Verification items for the finished model (mm, model axes). A direction names the side the tool comes from. Give positions to 0.01 mm unless a question says otherwise; leave off trailing zeros. Write each loop counter-clockwise with the first axis right and the second up, starting at its lowest first coordinate (ties: lowest second). Pieces come first, ordered by that corner, then holes.
from build123d import *
from build123d.topology import SkipClean

# Parameters (mm, degrees)
SKETCH1_R               = 19
BOSS_EXTRUDE1_DEPTH     = 5
BOSS_EXTRUDE4_DEPTH     = 20
SKETCH5_R               = 19
BOSS_EXTRUDE5_DEPTH     = 5
CUT_EXTRUDE1_DEPTH      = 37.701498607
CUT_EXTRUDE1_DEPTH_BACK = 5
SKETCH2_7_R             = 2.9
SKETCH1_3_R             = 9
CUT_EXTRUDE2_DEPTH      = 10
SKETCH6_R               = 2.5
BOSS_EXTRUDE7_DEPTH     = 25
FILLET1_R               = 5
SKETCH8_R               = 25
BOSS_EXTRUDE8_DEPTH     = 18


with BuildPart() as part:
    # Sketch1 → Boss-Extrude1 (new body)
    with BuildSketch(Plane(origin=(0, 0, 0), x_dir=(1, 0, 0), z_dir=(0, 1, 0))):
        with Locations(Location((0, 0, 0), (0, 0, 270))):
            Circle(SKETCH1_R)
    extrude(amount=BOSS_EXTRUDE1_DEPTH)

    # Sketch2 → Boss-Extrude4 (add)
    with SkipClean():  # the faces are left unmerged after this step: merging them gives an invalid solid
        with BuildSketch(Plane(origin=(0, 5, 0), x_dir=(1, 0, 0), z_dir=(0, 1, 0))):
            with BuildLine():
                Line((-14.008269399, 12.836213945), (-12.533714726, 11.485033529))
                ThreePointArc((-12.533714726, 11.485033529), (-12.02081528, 12.02081528), (-11.485033529, 12.533714726))
                Line((-11.485033529, 12.533714726), (-12.836213945, 14.008269399))
                ThreePointArc((-12.836213945, 14.008269399), (-13.435028843, 13.435028843), (-14.008269399, 12.836213945))
            make_face()
            with BuildLine():
                Line((14.008269399, 12.836213945), (12.533714726, 11.485033529))
                ThreePointArc((12.533714726, 11.485033529), (12.02081528, 12.02081528), (11.485033529, 12.533714726))
                Line((11.485033529, 12.533714726), (12.836213945, 14.008269399))
                ThreePointArc((12.836213945, 14.008269399), (13.435028843, 13.435028843), (14.008269399, 12.836213945))
            make_face()
            with BuildLine():
                Line((12.836213945, -14.008269399), (11.485033529, -12.533714726))
                ThreePointArc((11.485033529, -12.533714726), (12.02081528, -12.02081528), (12.533714726, -11.485033529))
                Line((12.533714726, -11.485033529), (14.008269399, -12.836213945))
                ThreePointArc((14.008269399, -12.836213945), (13.435028843, -13.435028843), (12.836213945, -14.008269399))
            make_face()
            with BuildLine():
                Line((-14.008269399, -12.836213945), (-12.533714726, -11.485033529))
                ThreePointArc((-12.533714726, -11.485033529), (-12.02081528, -12.02081528), (-11.485033529, -12.533714726))
                Line((-11.485033529, -12.533714726), (-12.836213945, -14.008269399))
                ThreePointArc((-12.836213945, -14.008269399), (-13.435028843, -13.435028843), (-14.008269399, -12.836213945))
            make_face()
        extrude(amount=BOSS_EXTRUDE4_DEPTH)

    # Sketch5 → Boss-Extrude5 (add)
    with SkipClean():  # the faces are left unmerged after this step: merging them gives an invalid solid
        with BuildSketch(Plane(origin=(0, 25, 0), x_dir=(1, 0, 0), z_dir=(0, 1, 0))):
            with Locations(Location((0, 0, 0), (0, 0, 270))):
                Circle(SKETCH5_R)
        extrude(amount=BOSS_EXTRUDE5_DEPTH)

    # Sketch2_7 → Cut-Extrude1 (cut, two sides: drawn at the far end of the back side and taken through both)
    with SkipClean():  # the faces are left unmerged after this step: merging them gives an invalid solid
        with BuildSketch(Plane(origin=(0, 5, 0), x_dir=(1, 0, 0), z_dir=(0, 1, 0)).offset(-CUT_EXTRUDE1_DEPTH_BACK)):
            with Locations(Location((14, 0, 0), (0, 0, 270))):
                Circle(SKETCH2_7_R)
            with Locations(Location((0, -14, 0), (0, 0, 270))):
                Circle(SKETCH2_7_R)
            with Locations(Location((0, 14, 0), (0, 0, 270))):
                Circle(SKETCH2_7_R)
            with Locations(Location((-14, 0, 0), (0, 0, 270))):
                Circle(SKETCH2_7_R)
        extrude(amount=CUT_EXTRUDE1_DEPTH + CUT_EXTRUDE1_DEPTH_BACK, mode=Mode.SUBTRACT)

    # Sketch1_3 → Cut-Extrude2 (cut)
    with SkipClean():  # the faces are left unmerged after this step: merging them gives an invalid solid
        with BuildSketch(Plane(origin=(0, 0, 0), x_dir=(1, 0, 0), z_dir=(0, 1, 0))):
            with Locations(Location((0, 0, 0), (0, 0, 270))):
                Circle(SKETCH1_3_R)
        extrude(amount=CUT_EXTRUDE2_DEPTH, mode=Mode.SUBTRACT)

    # Sketch6 → Boss-Extrude7 (add)
    with SkipClean():  # the faces are left unmerged after this step: merging them gives an invalid solid
        with BuildSketch(Plane(origin=(0, 30, 0), x_dir=(1, 0, 0), z_dir=(0, 1, 0))):
            with Locations(Location((0, 0, 0), (0, 0, 270))):
                Circle(SKETCH6_R)
        extrude(amount=BOSS_EXTRUDE7_DEPTH)

    # Fillet1
    fillet1_edges = [part.edges().sort_by_distance(p)[0] for p in [
        (0, 30, -2.5),
    ]]
    fillet(fillet1_edges, radius=FILLET1_R)

    # Sketch8 → Boss-Extrude8 (add)
    with SkipClean():  # the faces are left unmerged after this step: merging them gives an invalid solid
        with BuildSketch(Plane(origin=(0, 55, 0), x_dir=(1, 0, 0), z_dir=(0, 1, 0))):
            with Locations(Location((0, 0, 0), (0, 0, 270))):
                Circle(SKETCH8_R)
        extrude(amount=-BOSS_EXTRUDE8_DEPTH)


solid = part.part
Item 1: Sectioned sample at C-C on z = 16. Record the cut outline in (x, y).
Answer key:
outline: (-19.21, 37) - (19.21, 37) - (19.21, 55) - (-19.21, 55) - close; (-10.25, 0) - (-2.1, 0) - (-2.1, 5) - (-10.25, 5) - close; (-10.25, 25) - (-2.1, 25) - (-2.1, 30) - (-10.25, 30) - close; (2.1, 0) - (10.25, 0) - (10.25, 5) - (2.1, 5) - close; (2.1, 25) - (10.25, 25) - (10.25, 30) - (2.1, 30) - close
Item 2: Sectioned sample at B-B on y = 23.5. Record the cut outline in (x, z), then the cut area to 3 significant figures.
Answer key:
outline: (-14.01, -12.84) arc R19 ccw to (-12.84, -14.01) - (-11.49, -12.53) arc R17 cw to (-12.53, -11.49) - close; (-14.01, 12.84) - (-12.53, 11.49) arc R17 cw to (-11.49, 12.53) - (-12.84, 14.01) arc R19 ccw to start; (11.49, -12.53) - (12.84, -14.01) arc R19 ccw to (14.01, -12.84) - (12.53, -11.49) arc R17 cw to start; (11.49, 12.53) arc R17 cw to (12.53, 11.49) - (14.01, 12.84) arc R19 ccw to (12.84, 14.01) - close
area: 12.6 mm2
Item 3: Release check for a two-part mould opening along Z. For faces 1 (the face through (0.1, 2.5, -16.9)), 2 (the face through (-8, 30, 0)), 3 (the face through (12.17, 14.86, 13.28)), 4 (the face through (-13.28, 14.86, -12.17)) record: released by +Z, released by -Z, zero draft, split by the parting line, or undercut.
Answer key:
face 1: undercut
face 2: zero draft
face 3: released by +Z
face 4: undercut
Item 4: Sectioned sample at A-A on x = -15. Record the cut outline in (y, z).
Answer key:
outline: (0, -11.66) - (5, -11.66) - (5, -2.72) - (0, -2.72) - close; (0, 2.72) - (5, 2.72) - (5, 11.66) - (0, 11.66) - close; (25, -11.66) - (30, -11.66) - (30, -2.72) - (25, -2.72) - close; (25, 2.72) - (30, 2.72) - (30, 11.66) - (25, 11.66) - close; (37, -20) - (55, -20) - (55, 20) - (37, 20) - close
Item 5: Depth check by flat-ended pin: pin 1 (6 mm diameter, centred on y = 21, z = 2.5, fed in from +X); pin 2 (8 mm diameter, centred on y = 39.5, z = -14, fed in from -X); pin 3 (4.5 mm diameter, centred on x = 0, z = -14, fed in from -Y); pin 4 (1 mm diameter, centred on x = 16.5, y = 38, fed in from +Z). Enter the tip coordinate at first touch or a pass-through.
Answer key:
pin 1: passes through
pin 2: stops at x = -22.91
pin 3: stops at y = 37
pin 4: stops at z = 19.21
Item 6: Scan lines: line 1 along Z through (x, y) = (0, 4.05); line 2 along Y through (x, z) = (-8, 15). Record each from-to range of solid material in increasing order.
Answer key:
line 1: z = -19 to -16.9, -11.1 to -9, 9 to 11.1, 16.9 to 19
line 2: y = 0 to 5, 25 to 30, 37 to 55
Item 7: Sectioned sample at D-D on x = -10. Record the cut outline in (y, z).
Answer key:
outline: (0, -16.16) - (5, -16.16) - (5, 16.16) - (0, 16.16) - close; (25, -16.16) - (30, -16.16) - (30, 16.16) - (25, 16.16) - close; (37, -22.91) - (55, -22.91) - (55, 22.91) - (37, 22.91) - close
Item 8: Set-up check for faces 5 (the face through (0, 25, 0)), 6 (the face through (12.15, 14.86, -13.26)), 7 (the face through (-16.83, 27.46, -0.63)): record each of +Z, -Z, +X, -X, +Y, -Y from which the full face is reachable in a straight line by a thin tool's end or side.
Answer key:
face 5: none
face 6: -Z
face 7: -Y
